Solid Edge part; units mm, degrees
sketch "Sketch1" plane through (0, 0, 0) normal (0, 0, 1) x (1, 0, 0)
  circle A0 centre (-30.9705, 21.7021) radius 2.6
  line L0 (-16.4478, 31.2505) -> (-46.4478, 31.2505)
  line L1 (-46.4478, 31.2505) -> (-46.4478, 41.2505)
  line L2 (-46.4478, 41.2505) -> (-16.4478, 41.2505)
  line L3 (-16.4478, 41.2505) -> (-16.4478, 31.2505)
  circle A1 centre (-30.9705, 7.5433) radius 3.1
  circle A2 centre (50.8081, 24.0411) radius 2.9
  line L4 (72.3705, -6.0507) -> (-58.2724, -6.0507)
  line L5 (-58.2724, -6.0507) -> (-58.2724, 65.5066)
  line L6 (-58.2724, 65.5066) -> (72.3705, 65.5066)
  line L7 (72.3705, 65.5066) -> (72.3705, -6.0507)
  line L8 (30, 61.1519) -> (-30, 61.1519)
  line L9 (-30, 61.1519) -> (-30, 51.1519)
  line L10 (-30, 51.1519) -> (30, 51.1519)
  line L11 (30, 51.1519) -> (30, 61.1519)
  line L12 (57.0753, 31.058) -> (57.0753, 41.058)
  line L13 (57.0753, 41.058) -> (7.0753, 41.058)
  line L14 (7.0753, 41.058) -> (7.0753, 31.058)
  line L15 (7.0753, 31.058) -> (57.0753, 31.058)
  circle A3 centre (62.0753, 36.058) radius 1.75
  circle A4 centre (35, 56.1519) radius 1.75
  circle A5 centre (-51.4478, 36.2505) radius 1.75
  circle A6 centre (-35, 56.1519) radius 1.75
  circle A7 centre (2.0753, 36.058) radius 1.75
  circle A8 centre (-11.4478, 36.2505) radius 1.75
  circle A9 centre (13.4081, 4.8411) radius 2.9
  line L16 (48.3081, 6.9411) -> (48.3081, 22.0411)
  line L17 (48.3081, 22.0411) -> (18.0081, 22.0411)
  line L18 (18.0081, 22.0411) -> (18.0081, 6.9411)
  line L19 (18.0081, 6.9411) -> (48.3081, 6.9411)
  circle A10 centre (13.4081, 24.0411) radius 2.9
  circle A11 centre (50.8081, 4.8411) radius 2.9
extrude "Protrusion1" add sketch "Sketch1" along normal blind 2
fillet "Round_1" [suppressed]
fillet "Round_2" [suppressed]
sketch "Sketch2" plane through (0, 0, 0) normal (0, 0, 1) x (1, 0, 0)
  circle A0 centre (-30.9992, 16.4354) radius 1.5
  circle A1 centre (-30.9992, 16.4354) radius 1.9
extrude "ExtrudedProtrusion_3" add sketch "Sketch2" against normal blind 1.1
fillet "Round_3" radius 5 4 edges at (-58.2724, -6.0507, 1) (-58.2724, 65.5066, 1) (72.3705, -6.0507, 1) (72.3705, 65.5066, 1)
fillet "Round_4" radius 1 8 edges at (7.049, 65.5066, 2) (70.906, 64.0422, 2) (72.3705, 29.7279, 2) (70.906, -4.5863, 2) (7.049, -6.0507, 2) (-56.8079, -4.5863, 2) (-58.2724, 29.7279, 2) (-56.8079, 64.0422, 2)
sketch "Sketch3" plane through (0, 0, 0) normal (0, 0, 1) x (1, 0, 0)
  circle A0 centre (50.8081, 4.8411) radius 2.9
  circle A1 centre (13.4081, 4.8411) radius 2.9
  circle A2 centre (13.4081, 24.0411) radius 2.9
  circle A3 centre (50.8081, 24.0411) radius 2.9
extrude "ExtrudedProtrusion_6" add sketch "Sketch3" along normal blind 2
sketch "Sketch4" plane through (0, 0, 0) normal (0, 0, 1) x (1, 0, 0)
  circle A0 centre (50.8081, 24.0411) radius 2.9
  circle A1 centre (50.8081, 24.0411) radius 1.45
  circle A2 centre (50.8081, 4.8411) radius 2.9
  circle A3 centre (50.8081, 4.8411) radius 1.45
  circle A4 centre (13.4081, 4.8411) radius 2.9
  circle A5 centre (13.4081, 4.8411) radius 1.45
  circle A6 centre (13.4081, 24.0411) radius 2.9
  circle A7 centre (13.4081, 24.0411) radius 1.45
extrude "ExtrudedProtrusion_7" add sketch "Sketch4" against normal blind 6
Work out the finished part from the listing and answer in its coordinate system (mm). A direction names the side the tool comes from. Give positions to 0.01 mm unless a question says otherwise; leave off trailing zeros. Loops run counter-clockwise (first coordinate to the right, second up) from the corner with the lowest first, then second, coordinate; pieces in that order, holes last. Notation, with made-up numbers: (-14, -17.5) - (40, -17.5) arc R30 ccw to (40, 17.5) - close; hole circle Ø5 at (19.25, -30.75). An arc over 180 degrees is marked (long way). Use CSV: the item, a comma, the result in double quotes. Start each with the question number.
(1) Each of these flat-tipped pins is pushed along its axis until it touches: pin 1 (1 mm diameter, centred on y = 24.5, z = -2, fed in from -X); pin 2 (1.6 mm diameter, centred on x = -32, z = 1.5, fed in from -Y); pin 3 (1 mm diameter, centred on x = -19.5, y = 25.5, fed in from -Z); pin 4 (0.6 mm diameter, centred on x = -7, z = 1.5, fed in from +Y). Where does it stop, or does it pass through?
(2) Find the intervals of material crossed by L1, parallel to Y at x = -25, z = 1; L2, parallel to X at y = 12, z = 0.75; L3, parallel to Y at x = -7.5, z = 0.5, in increasing order.
(3) Find section C-C, the plane x = 9. Determine the outline of the cut face in (y, z).
(4) Find section A-A, the plane x = 40. Determine the outline of the cut face in (y, z).
(5) Find section D-D, the plane y = 29. Determine the outline of the cut face in (x, z).
(6) Find section B-B, the plane z = -3. Determine the outline of the cut face in (x, y), plus the area to 3 significant figures.
(7) Determine the mould class of faces 1 (the face through (49, 4, -6)), 2 (the face through (70.945, 64.003, 0.507)), 3 (the face through (10.51, 4.97, -2.96)) for opening direction Y: released by +Y, released by -Y, zero draft, split by the parting line, or undercut.
(8) A tool of negligible diameter and unlimited length cuts with its end or side. For faces 4 (the face through (8, 30, 2)), 5 (the face through (-31, 16, 0)), from which of +Z, -Z, +X, -X, +Y, -Y can it reach the whole face along a straight path? Write none if from no direction.
Results found:
1,pin 1,"x = 10.51"
1,pin 2,"y = -6.05"
1,pin 3,"z = 0"
1,pin 4,"y = 65.49"
2,L1,"-6.05 to 31.25, 41.25 to 51.15, 61.15 to 65.51"
2,L2,"-58.27 to 18.01, 48.31 to 72.37"
2,L3,"-6.05 to 51.15, 61.15 to 65.51"
3,outline,"(-6.05, 0) - (31.06, 0) - (31.06, 2) - (-5.05, 2) arc R1 ccw to (-6.05, 1) - close; (41.06, 0) - (51.15, 0) - (51.15, 2) - (41.06, 2) - close; (61.15, 0) - (65.51, 0) - (65.51, 1) arc R1 ccw to (64.51, 2) - (61.15, 2) - close"
4,outline,"(-6.05, 0) - (6.94, 0) - (6.94, 2) - (-5.05, 2) arc R1 ccw to (-6.05, 1) - close; (22.04, 0) - (31.06, 0) - (31.06, 2) - (22.04, 2) - close; (41.06, 0) - (65.51, 0) - (65.51, 1) arc R1 ccw to (64.51, 2) - (41.06, 2) - close"
5,outline,"(-58.27, 0) - (72.37, 0) - (72.37, 1) arc R1 ccw to (71.37, 2) - (-57.27, 2) arc R1 ccw to (-58.27, 1) - close"
6,outline,"circle Ø5.8 at (13.41, 4.84); circle Ø5.8 at (13.41, 24.04); circle Ø5.8 at (50.81, 4.84); circle Ø5.8 at (50.81, 24.04); hole circle Ø2.9 at (13.41, 4.84); hole circle Ø2.9 at (13.41, 24.04); hole circle Ø2.9 at (50.81, 4.84); hole circle Ø2.9 at (50.81, 24.04)"
6,area,"79.3 mm^2"
7,face 1,"zero draft"
7,face 2,"released by +Y"
7,face 3,"undercut"
8,face 4,"+Z, +X, -X, +Y, -Y"
8,face 5,"-Z"
